Check sheet for the modelled part. Datum: model origin and axes. Units: mm. A direction names the side the tool comes from. Give positions to 0.01 mm unless a question says otherwise; leave off trailing zeros. Loops run counter-clockwise (first coordinate to the right, second up) from the corner with the lowest first, then second, coordinate; pieces in that order, holes last. Notation, with made-up numbers: M -15,9.25 L 15,9.25 A18 cw 15,29.25 Z; hole C -4,-23.5 d3. An arc over 180 degrees is marked long. Write each question's results on one line, items separated by ' | '. Start each with the question number.
1. Sectioned sample at A-A on x = 129. Record the cut outline in (y, z), and give its area (3 significant figures).
2. Sectioned sample at D-D on z = 0.9. Give the number of separate pieces and of enclosed holes in the cut face, and give its area (3 significant figures).
3. Material ranges on line 1 along X through (y, z) = (-23.5, 0.45); line 2 along X through (y, z) = (6.5, 1.4); line 3 along Y through (x, z) = (43, 0.9), recorded low to high.
4. Draft check along X on faces 5 (the flat face through (-6.065, -13.672, 1.479)), 6 (the cylindrical face through (186.9, 26.2, 1.5)), 7 (the cylindrical face through (187.743, -25.481, 1.521)), 8 (the cylindrical face through (181.291, -4.793, 1.479)). Enter one of: pulls with the +X half, pulls with the -X half, needs draft (parallel to the pull), parting line crosses it, or undercut.
5. Sectioned sample at B-B on y = 0. Record the cut outline in (x, z).
6. Tool access check on faces 1 (the flat face through (28.071, -17.436, 1.479)), 2 (the flat face through (105, -2, 3)), 3 (the cylindrical face through (165.09, -18.17, 1.48)), 4 (the cylindrical face through (120.416, 2.703, 2.507)). Record the directions out of +Z, -Z, +X, -X, +Y, -Y that give a thin tool (end or side, any length) a straight path to the whole face; none if there is none.
7. Go/stop test with flat-tipped pins: pin 1 (3.5 mm diameter, centred on x = 183.23, y = -16.84, fed in from +Z); pin 2 (0.5 mm diameter, centred on y = -17, z = 2, fed in from -X); pin 3 (0.9 mm diameter, centred on x = 145, z = 1, fed in from +Y). Record where each tip stops, or that it passes through.
8. Sectioned sample at C-C on x = 43. Record the cut outline in (y, z).
```python
from build123d import *

# Parameters (mm, degrees)
SKETCH_1_R          = 8
EXTRUDE_1_DEPTH     = 3
HOLE_WIZARD_M31_D   = 3.4
HOLE_WIZARD_M51_D   = 5.5
HOLE_WIZARD_M52_D   = 5.5
FILLET_1_R          = 10
FILLET_2_R          = 5
CUT_EXTRUDE_1_DEPTH = 195.061830596
FILLET_3_R          = 4
SKETCH_9_R          = 9
CUT_EXTRUDE_2_DEPTH = 1


with BuildPart() as part:
    # Эскиз1 → Бобышка-Вытянуть1 (new body)
    with BuildSketch(Plane.XY):
        with BuildLine():
            Line((-9.508526364, -3.096437692), (-1.398717752, -28))
            Line((-1.398717752, -28), (189.947361129, -28))
            ThreePointArc((189.947361129, -28), (191.995297124, 1.34383112), (189.536809823, 30.656120467))
            Line((189.536809823, 30.656120467), (125.388049295, 13.526041997))
            ThreePointArc((125.388049295, 13.526041997), (123.105499175, 12.698616461), (121.000225207, 11.489282104))
            Line((121.000225207, 11.489282104), (83.76563687, -14.436473614))
            Line((83.76563687, -14.436473614), (63.718090084, -22))
            Line((63.718090084, -22), (35.731449132, -22))
            Line((35.731449132, -22), (20.675178874, -13.02912429))
            Line((20.675178874, -13.02912429), (8.326583423, 5.537870395))
            ThreePointArc((8.326583423, 5.537870395), (-4.357415095, 9.00071851), (-9.508526364, -3.096437692))
        make_face()
        with Locations((129, 0)):
            Circle(SKETCH_1_R, mode=Mode.SUBTRACT)
    extrude(amount=EXTRUDE_1_DEPTH)

    # Отверстие с зазором M31 (through all)
    with Locations(Plane.XY.offset(3)):
        with Locations((9, -25), (43, -25), (77, -25)):
            Hole(HOLE_WIZARD_M31_D / 2)

    # Отверстие с зазором M51 (through all)
    with Locations(Plane.XY.offset(3)):
        with Locations((0, 0)):
            Hole(HOLE_WIZARD_M51_D / 2)

    # Отверстие с зазором M52 (through all)
    with Locations(Plane.XY.offset(3)):
        with Locations((183.228106674, 16.836297834), (183.914180714, 5.619086431), (183.914180714, -5.619086431), (183.228106674, -16.836297834)):
            Hole(HOLE_WIZARD_M52_D / 2)

    # Скругление1
    fillet_1_edges = [part.edges().sort_by_distance(p)[0] for p in [
        (35.731449132, -22, 1.5),
        (63.718090084, -22, 1.5),
        (83.76563687, -14.436473614, 1.5),
        (189.536809823, 30.656120467, 1.5),
        (189.947361129, -28, 1.5),
        (20.675178874, -13.02912429, 1.5),
    ]]
    fillet(fillet_1_edges, radius=FILLET_1_R)

    # Скругление2
    fillet_2_edges = [part.edges().sort_by_distance(p)[0] for p in [
        (-1.398717752, -28, 1.5),
    ]]
    fillet(fillet_2_edges, radius=FILLET_2_R)

    # Эскиз8 → Вырез-Вытянуть1 (cut, through all)
    with BuildSketch(Plane.XY.offset(3)):
        with BuildLine():
            Line((138.90792063, 9.891062066), (175.404223108, 19.636917172))
            ThreePointArc((175.404223108, 19.636917172), (176.470620047, 3.220288824), (176.003884761, -13.22431658))
            Line((176.003884761, -13.22431658), (138.90792063, 9.891062066))
        make_face()
        with BuildLine():
            Line((142.971746687, -0.888985098), (175.246255309, -21))
            Line((175.246255309, -21), (132.5, -21))
            Line((132.5, -21), (132.5, -13.555441712))
            ThreePointArc((132.5, -13.555441712), (139.790053932, -8.92046726), (142.971746687, -0.888985098))
        make_face()
        with BuildLine():
            Line((115.05010243, -1.183367143), (86.589440581, -21))
            Line((86.589440581, -21), (125.5, -21))
            Line((125.5, -21), (125.5, -13.555441712))
            ThreePointArc((125.5, -13.555441712), (118.304590303, -9.033726331), (115.05010243, -1.183367143))
        make_face()
    extrude(amount=-CUT_EXTRUDE_1_DEPTH, mode=Mode.SUBTRACT)

    # Скругление3
    fillet_3_edges = [part.edges().sort_by_distance(p)[0] for p in [
        (175.404223108, 19.636917172, 1.5),
        (176.003884761, -13.22431658, 1.5),
        (138.90792063, 9.891062066, 1.5),
        (115.05010243, -1.183367143, 1.5),
        (125.5, -13.555441712, 1.5),
        (125.5, -21, 1.5),
        (86.589440581, -21, 1.5),
        (175.246255309, -21, 1.5),
        (132.5, -21, 1.5),
        (132.5, -13.555441712, 1.5),
        (142.971746687, -0.888985098, 1.5),
    ]]
    fillet(fillet_3_edges, radius=FILLET_3_R)

    # Эскиз9 → Вырез-Вытянуть2 (cut)
    with BuildSketch(Plane(origin=(0, 0, 3), x_dir=(-1, 0, 0), z_dir=(0, 0, -1))):
        with Locations((-129, 0)):
            Circle(SKETCH_9_R)
    extrude(amount=CUT_EXTRUDE_2_DEPTH, mode=Mode.SUBTRACT)


solid = part.part
```
Output values:
1) outline: M -28,0 L -8,0 L -8,2 L -9,2 L -9,3 L -28,3 Z; M 8,0 L 14.49,0 L 14.49,3 L 9,3 L 9,2 L 8,2 Z | area: 77.5 mm2
2) separate pieces: 1 | enclosed holes: 12 | area: 4,120 mm2
3) line 1: -2.86 to 8.2, 9.8 to 42.2, 43.8 to 76.2, 77.8 to 189.46 | line 2: -7.6 to 7.6, 113.83 to 124.34, 133.66 to 145.34, 176.38 to 181.31, 186.52 to 191.89 | line 3: -28 to -26.7, -23.3 to -22
4) face 5: pulls with the -X half | face 6: parting line crosses it | face 7: pulls with the +X half | face 8: undercut
5) outline: M -10,0 L -2.75,0 L -2.75,3 L -10,3 Z; M 2.75,0 L 12.01,0 L 12.01,3 L 2.75,3 Z; M 104.5,0 L 121,0 L 121,2 L 120,2 L 120,3 L 104.5,3 Z; M 137,0 L 154.78,0 L 154.78,3 L 138,3 L 138,2 L 137,2 Z; M 176.5,0 L 192,0 L 192,3 L 176.5,3 Z
6) face 1: +Z, -Z, +Y | face 2: +Z, +X, -X, +Y, -Y | face 3: +Z, -Z | face 4: +Z
7) pin 1: through | pin 2: x = -5.06 | pin 3: y = 18.88
8) outline: M -28,0 L -26.7,0 L -26.7,3 L -28,3 Z; M -23.3,0 L -22,0 L -22,3 L -23.3,3 Z
